from build123d import *

# Parameters (mm, degrees)
F1_DEPTH     = 70
F2_T         = 4
F3_T1_DEPTH  = 774.9998275448
F3_T3_DEPTH  = 114.9996550895
F3_T6_ANGLE  = 90.0000000944
F3_T8_ANGLE  = 89.9999999363
F3_T10_ANGLE = 90.0000000944
F3_T12_ANGLE = 89.9999999363
F4_R         = 15
F5_DEPTH     = 70.001


# Not quite as in the source:
# - a fillet or chamfer that OpenCascade refuses, or shapes differently, is made with other operations: its cross-section is extruded or revolved along the edge and cut away or added
# - a shell that OpenCascade refuses in one call is made with other operations: the cavity is built on its own and cut out


with BuildPart() as f1:
    # F0 (on Front) → F1 (new body)
    with BuildSketch(Plane.XZ):
        with BuildLine():
            Line((-374.9998275448, -45), (375, -45))
            Line((375, -45), (375, 45))
            Line((375, 45), (-374.9998275448, 45))
            ThreePointArc((-374.9998275448, 45), (-374.999949489, 44.999949489), (-375, 44.9998275448))
            Line((-375, 44.9998275448), (-375, -44.9998275448))
            ThreePointArc((-375, -44.9998275448), (-374.999949489, -44.999949489), (-374.9998275448, -45))
        make_face()
    extrude(amount=F1_DEPTH)

    # F2: shell of thickness 4, made by hand


with BuildPart() as f2_core1:
    # F2_t2: copy of F1
    add(f1.part)

    # the walls: a layer under each face that stays
    f2_faces = [f2_core1.faces().sort_by_distance(p)[0] for p in [
        (8.62276e-05, -35, -45),
        (8.62276e-05, -35, 45),
        (0, 0, 0),
        (0, -70, 0),
    ]]
    thicken(f2_faces, amount=-F2_T, mode=Mode.SUBTRACT)


with BuildPart() as f1_1:
    add(f1.part)

    # what is left inside the walls is the cavity
    f2_cavity = [f2_core1.part.solids().sort_by_distance(p)[0] for p in [
        (0, -4.04, -15),
    ]]
    add(f2_cavity, mode=Mode.SUBTRACT)

    # F3: fillet of radius 5 on 4 edges, made by hand

    # F3_s2 → F3_t1 (cut)
    with BuildSketch(Plane.YZ.offset(-387.4998275448)):
        with BuildLine():
            ThreePointArc((-70, 40), (-68.5355339059, 43.5355339059), (-65, 45))
            Line((-65, 45), (-70, 45))
            Line((-70, 45), (-70, 40))
        make_face()
        with BuildLine():
            ThreePointArc((0, 40), (-1.4644660941, 43.5355339059), (-5, 45))
            Line((-5, 45), (0, 45))
            Line((0, 45), (0, 40))
        make_face()
        with BuildLine():
            ThreePointArc((-5, -45), (-1.4644660941, -43.5355339059), (0, -40))
            Line((0, -40), (0, -45))
            Line((0, -45), (-5, -45))
        make_face()
        with BuildLine():
            ThreePointArc((-65, -45), (-68.5355339059, -43.5355339059), (-70, -40))
            Line((-70, -40), (-70, -45))
            Line((-70, -45), (-65, -45))
        make_face()
    extrude(amount=F3_T1_DEPTH, mode=Mode.SUBTRACT)

    # F3_s4 → F3_t3 (cut)
    with BuildSketch(Plane.XY.offset(-57.4998275448)):
        with BuildLine():
            ThreePointArc((-370, -70), (-373.5355339059, -68.5355339059), (-375, -65))
            Line((-375, -65), (-375, -70))
            Line((-375, -70), (-370, -70))
        make_face()
        with BuildLine():
            ThreePointArc((-370, 0), (-373.5355339059, -1.4644660941), (-375, -5))
            Line((-375, -5), (-375, 0))
            Line((-375, 0), (-370, 0))
        make_face()
    extrude(amount=F3_T3_DEPTH, mode=Mode.SUBTRACT)

    # F3_s5 → F3_t6 (revolve, cut)
    with BuildSketch(Plane.XY.offset(-44.9998275448)):
        with BuildLine():
            ThreePointArc((-375, -65), (-374.999956886, -65.0207638646), (-374.9998275448, -65.0415273711))
            Line((-374.9998275448, -65.0415273711), (-374.9998275448, -70))
            Line((-374.9998275448, -70), (-375, -70))
            Line((-375, -70), (-375, -65))
        make_face()
    revolve(axis=Axis((-374.9998275448, -70, -44.9998275448), (0, -1, 0)), revolution_arc=F3_T6_ANGLE, mode=Mode.SUBTRACT)

    # F3_s7 → F3_t8 (revolve, cut)
    with BuildSketch(Plane.YZ.offset(-374.9998275448)):
        with BuildLine():
            ThreePointArc((-65.0415273711, 44.9998275448), (-65.0207638646, 44.999956886), (-65, 45))
            Line((-65, 45), (-70, 45))
            Line((-70, 45), (-70, 44.9998275448))
            Line((-70, 44.9998275448), (-65.0415273711, 44.9998275448))
        make_face()
    revolve(axis=Axis((-374.9998275448, -70, 44.9998275448), (0, -1, 0)), revolution_arc=F3_T8_ANGLE, mode=Mode.SUBTRACT)

    # F3_s9 → F3_t10 (revolve, cut)
    with BuildSketch(Plane.XY.offset(-44.9998275448)):
        with BuildLine():
            ThreePointArc((-375, -5), (-374.999956886, -4.9792361354), (-374.9998275448, -4.9584726289))
            Line((-374.9998275448, -4.9584726289), (-374.9998275448, 0))
            Line((-374.9998275448, 0), (-375, 0))
            Line((-375, 0), (-375, -5))
        make_face()
    revolve(axis=Axis((-374.9998275448, 0, -44.9998275448), (0, -1, 0)), revolution_arc=F3_T10_ANGLE, mode=Mode.SUBTRACT)

    # F3_s11 → F3_t12 (revolve, cut)
    with BuildSketch(Plane.YZ.offset(-374.9998275448)):
        with BuildLine():
            ThreePointArc((-4.9584726289, 44.9998275448), (-4.9792361354, 44.999956886), (-5, 45))
            Line((-5, 45), (0, 45))
            Line((0, 45), (0, 44.9998275448))
            Line((0, 44.9998275448), (-4.9584726289, 44.9998275448))
        make_face()
    revolve(axis=Axis((-374.9998275448, 0, 44.9998275448), (0, -1, 0)), revolution_arc=F3_T12_ANGLE, mode=Mode.SUBTRACT)

    # F4 (on Front) → F5 (cut, through all)
    with BuildSketch(Plane.XZ):
        with Locations((302, -5)):
            Circle(F4_R)
    extrude(amount=F5_DEPTH, mode=Mode.SUBTRACT)


solid = f1_1.part
Can you work these out from the model? Positions are in its coordinate system, mm. A direction names the side the tool comes from. Give positions to 0.01 mm unless a question says otherwise; leave off trailing zeros. Order: outer loops, then holes, each group sorted by start corner. A loop starts at its lowest first (then second) coordinate and runs counter-clockwise, first axis right, second up. Notation, with made-up numbers: M 74,-15.5 L 102,-15.5 A29 ccw 102,22.5 Z; hole C -13,-11.5 d11. An arc over 180 degrees is marked long. Use a Markdown table: item, result. Add a question column.
Item 1: Suppose I cut it at D-D (x = -33.5). List the corners of the cut face in (y, z) for me, then the cut area to 3 significant figures.
Item 2: If I drill on L1, parallel to Z at x = 257, y = -20.5; L2, parallel to Y at x = -138.5, z = 0; L3, parallel to Z at x = 302, y = -67, over which ranges is the centre line in solid material (lowest first)? Write a range as [from, to].
Item 3: For faces 4 (the cylindrical face through (315.856, -1.972, -10.745)), 5 (the flat face through (-5, -35, -41)), which set-ups out of +Z, -Z, +X, -X, +Y, -Y let a thin tool reach every point of the face, with its end or its side?
Item 4: We'd pull the mould along Z, two halves only. Please class faces 1 (the flat face through (5, -35, 45)), 2 (the flat face through (375, -3.7, -0.2)), 3 (the flat face through (-5, -66, 1)): +Z half, -Z half, draft (parallel to the pull), parting line (faces both ways), or undercut.
Item 5: Suppose I cut it at B-B (y = -47.5). List the corners of the cut face in (x, z) for me.
Item 6: Suppose I cut it at C-C (z = -5). List the corners of the cut face in (x, y) for me, then the cut area to 3 significant figures.
Item 7: Suppose I cut it at A-A (x = 302). List the corners of the cut face in (y, z) for me.
Answer sheet:
| question | item | result |
|---|---|---|
| 1 | outline | M -70,-40 A5 ccw -65,-45 L -5,-45 A5 ccw 0,-40 L 0,40 A5 ccw -5,45 L -65,45 A5 ccw -70,40 Z; hole M -66,-41 L -4,-41 L -4,41 L -66,41 Z |
| 1 | area | 1,190 mm² |
| 2 | L1 | z = [-45, -41], [41, 45] |
| 2 | L2 | y = [-70, -66], [-4, 0] |
| 2 | L3 | z = [-44.58, -20], [10, 44.58] |
| 3 | face 4 | +Y, -Y |
| 3 | face 5 | +X, -X |
| 4 | face 1 | +Z half |
| 4 | face 2 | draft |
| 4 | face 3 | undercut |
| 5 | outline | M -375,-45 L 375,-45 L 375,-41 L -375,-41 Z; M -375,41 L 375,41 L 375,45 L -375,45 Z |
| 6 | outline | M -374.9,-66 A5 ccw -370,-70 L 287,-70 L 287,-66 Z; M -374.9,-4 L 287,-4 L 287,0 L -370,0 A5 ccw Z; M 317,-70 L 375,-70 L 375,-66 L 317,-66 Z; M 317,-4 L 375,-4 L 375,0 L 317,0 Z |
| 6 | area | 5,750 mm² |
| 7 | outline | M -70,-40 A5 ccw -65,-45 L -5,-45 A5 ccw 0,-40 L 0,-20 L -4,-20 L -4,-41 L -66,-41 L -66,-20 L -70,-20 Z; M -70,10 L -66,10 L -66,41 L -4,41 L -4,10 L 0,10 L 0,40 A5 ccw -5,45 L -65,45 A5 ccw -70,40 Z |
